Read the model definition and answer for the solid it produces. Units are mm, in the model's axes. Face numbers are marked on the shaded views. A direction names the side the tool comes from. Round coordinates to 2 decimals unless told otherwise and drop trailing zeros. Order: outer loops, then holes, each group sorted by start corner. A loop starts at its lowest first (then second) coordinate and runs counter-clockwise, first axis right, second up. Notation, with made-up numbers: (38.25, 33) -> (96.25, 33) arc R18 cw to (96.25, 63) -> close; hole circle Ø2 at (3, -24). An arc over 180 degrees is marked (long way). Use a Markdown table: item, result. Add a question column.
1. The mould has two halves that part along Y. Classify the marked faces 1 and 2: +Y half, -Y half, draft (parallel to the pull), parting line (faces both ways), or undercut.
2. Given pin 1 (4 mm diameter, centred on y = 24, z = -1.5, fed in from +X); pin 2 (3 mm diameter, centred on x = -6, z = -7.5, fed in from +Y); pin 3 (12 mm diameter, centred on x = -2.5, z = -4, fed in from +Y); pin 4 (8 mm diameter, centred on x = 9, y = 22, fed in from -Z), each flat-ended and moving along its own axis, determine where each tip first touches the part or whether it passes through.
3. Section A-A, the plane y = 17.5 is taken. Give the vertices of the cut face in (x, z), then the cut area to 3 significant figures.
4. Consider L1, parallel to Y at x = 11.25, z = -2.75; L2, parallel to Y at x = 4.75, z = -11.75; L3, parallel to X at y = 24.5, z = -0.5. Determine where each line is inside the solid, lowest interval first. Write a range as [from, to].
5. For the marked faces 3, 4 and 5, determine the directions among +Z, -Z, +X, -X, +Y, -Y from which every point of the face is accessible in a straight line to the end or side of a thin tool.
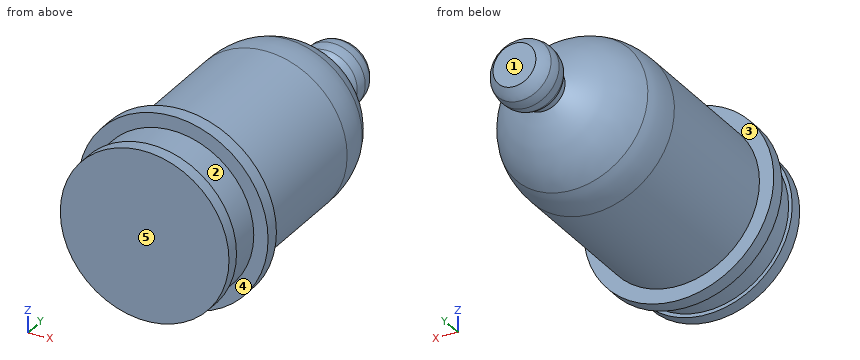
```python
from build123d import *

# Parameters (mm, degrees)
SKETCH1_R           = 11.8
BOSS_EXTRUDE1_DEPTH = 1.8
SKETCH2_R           = 11.3
BOSS_EXTRUDE2_DEPTH = 5
SKETCH3_R           = 13.3
BOSS_EXTRUDE3_DEPTH = 2
SKETCH4_R           = 11.3
BOSS_EXTRUDE4_DEPTH = 20.4
SKETCH6_R           = 3
BOSS_EXTRUDE5_DEPTH = 1


with BuildPart() as part:
    # Sketch1 → Boss-Extrude1 (new body)
    with BuildSketch(Plane(origin=(0, 0, 0), x_dir=(1, 0, 0), z_dir=(0, 1, 0))):
        Circle(SKETCH1_R)
    extrude(amount=BOSS_EXTRUDE1_DEPTH)

    # Sketch2 → Boss-Extrude2 (add)
    with BuildSketch(Plane(origin=(0, 1.8, 0), x_dir=(1, 0, 0), z_dir=(0, 1, 0))):
        Circle(SKETCH2_R)
    extrude(amount=BOSS_EXTRUDE2_DEPTH)

    # Sketch3 → Boss-Extrude3 (add)
    with BuildSketch(Plane(origin=(0, 6.8, 0), x_dir=(1, 0, 0), z_dir=(0, 1, 0))):
        Circle(SKETCH3_R)
    extrude(amount=BOSS_EXTRUDE3_DEPTH)

    # Sketch4 → Boss-Extrude4 (add)
    with BuildSketch(Plane(origin=(0, 8.8, 0), x_dir=(1, 0, 0), z_dir=(0, 1, 0))):
        Circle(SKETCH4_R)
    extrude(amount=BOSS_EXTRUDE4_DEPTH)

    # Sketch5 → Revolve1 (revolve)
    with BuildSketch(Plane(origin=(0, 0, 0), x_dir=(0, 0, -1), z_dir=(1, 0, 0))):
        with BuildLine():
            add(Edge.make_bspline(
                [(-10.5, 34.2), (-8.718155673, 38.74792404), (-3, 41.2)],
                knots=[0.330462847, 0.330462847, 0.330462847, 1, 1, 1], degree=2))
            Line((-10.5, 34.2), (0, 34.2))
            Line((0, 34.2), (0, 41.2))
            Line((0, 41.2), (-3, 41.2))
        make_face()
        with BuildLine():
            add(Edge.make_bspline(
                [(-11.3, 29.2), (-11.379463292, 31.955285248), (-10.5, 34.2)],
                knots=[0, 0, 0, 0.330462847, 0.330462847, 0.330462847], degree=2))
            Line((-11.3, 29.2), (0, 29.2))
            Line((0, 29.2), (0, 34.2))
            Line((0, 34.2), (-10.5, 34.2))
        make_face()
    revolve(axis=Axis((0, 29.2, 0), (0, 1, 0)))

    # Sketch6 → Boss-Extrude5 (add)
    with BuildSketch(Plane(origin=(0, 41.2, 0), x_dir=(1, 0, 0), z_dir=(0, 1, 0))):
        Circle(SKETCH6_R)
    extrude(amount=BOSS_EXTRUDE5_DEPTH)

    # Sketch7 → Revolve2 (revolve)
    with BuildSketch(Plane(origin=(0, 0, 0), x_dir=(0, 0, -1), z_dir=(1, 0, 0))):
        with BuildLine():
            Line((-4.25, 43.7), (0, 43.7))
            Line((0, 43.7), (0, 45.2))
            Line((0, 45.2), (-4.5, 45.2))
            add(Edge.make_bspline(
                [(-4.25, 43.7), (-4.53338952, 44.377370072), (-4.5, 45.2)],
                knots=[0.56217108, 0.56217108, 0.56217108, 1, 1, 1], degree=2))
        make_face()
        with BuildLine():
            Line((-3, 42.2), (0, 42.2))
            Line((0, 42.2), (0, 43.7))
            Line((0, 43.7), (-4.25, 43.7))
            add(Edge.make_bspline(
                [(-3, 42.2), (-3.886128668, 42.830258767), (-4.25, 43.7)],
                knots=[0, 0, 0, 0.56217108, 0.56217108, 0.56217108], degree=2))
        make_face()
    revolve2 = revolve(axis=Axis((0, 42.2, 0), (0, 1, 0)))

    # Mirror1: Revolve2 across plane
    add(revolve2.mirror(Plane(origin=(0, 45.2, 0), x_dir=(0, 0, 1), z_dir=(0, -1, 0))))


solid = part.part
```
Verdict:
| question | item | result |
|---|---|---|
| 1 | face 1 | +Y half |
| 1 | face 2 | undercut |
| 2 | pin 1 | stops at x = 11.3 |
| 2 | pin 2 | stops at y = 37.86 |
| 2 | pin 3 | stops at y = 48.2 |
| 2 | pin 4 | stops at z = -10.13 |
| 3 | outline | circle Ø22.6 at (0, 0) |
| 3 | area | 401 mm2 |
| 4 | L1 | y = [0, 1.8], [6.8, 8.8] |
| 4 | L2 | y = [6.8, 8.8] |
| 4 | L3 | x = [-11.29, 11.29] |
| 5 | face 3 | +Y |
| 5 | face 4 | none |
| 5 | face 5 | +Z, -Z, +X, -X, -Y |
